Part model, mm, in its own coordinate system. Give positions to 0.01 mm unless a question says otherwise; leave off trailing zeros. Write each loop counter-clockwise with the first axis right and the second up, starting at its lowest first coordinate (ties: lowest second). Pieces come first, ordered by that corner, then holes. Notation, with made-up numbers: M 36.5,37.25 L 84.5,37.25 A23 ccw 84.5,68.25 Z; hole C 75.25,-2 d10. An arc over 180 degrees is marked long. Use CSV: the item, a comma, the result in double quotes. Start each with the question number.
Item 1: Cut at A-A (z = 46). List the corners of the cut face in (x, y), then the cut area to 3 significant figures.
Item 2: Mould opens along Y. For faces 1 (the flat face through (0, -1.23, 47.34)), 2 (the flat face through (5, -5.2, 47)), 3 (the cylindrical face through (4.93, -0.496, 44.425)) say: released by +Y, released by -Y, zero draft, split by the parting line, or undercut.
Item 3: Cut at C-C (x = 4.5). List the corners of the cut face in (y, z).
Item 4: Pin check, flat tip, straight feed: pin 1 (5 mm diameter, centred on x = 3.5, y = 3, fed in from -Z). Stop position of the tip, or through.
Item 5: Cut at D-D (x = 9.25). List the corners of the cut face in (y, z), then the cut area to 3 significant figures.
Item 6: Drill centre lines: line 1 (Y direction, x = 7.5, z = 46); line 2 (Z direction, x = 2.75, y = -1.5); line 3 (Z direction, x = 6.75, y = 0). Where is each one in solid material? Low to high. Write a range as [from, to].
Item 7: Cut at B-B (y = 0). List the corners of the cut face in (x, z), then the cut area to 3 significant figures.
Autodesk Inventor part; units mm, degrees
ref_plane "YZ Plane" through (0, 0, 0) normal (1, 0, 0) x (0, 1, 0)
ref_plane "XZ Plane" through (0, 0, 0) normal (0, 1, 0) x (-1, 0, 0)
ref_plane "XY Plane" through (0, 0, 0) normal (0, 0, 1) x (1, 0, 0)
sketch "Sketch1" plane through (0, 0, 0) normal (1, 0, 0) x (0, 1, 0)
  circle A0 centre (0, 0) radius 54
  circle A1 centre (0, 46) radius 1
  circle A2 centre (0, 46) radius 5.5
  line L0 (5.2, 40.5) -> (-5.2, 40.5)
  arc A3 (5.2, 53.749) -> (-5.2, 53.749) centre (0, 0) ccw
  line L1 (5.2, 53.749) -> (5.2, 40.5)
  line L2 (-5.2, 53.749) -> (-5.2, 40.5)
  circle A4 centre (0, 46) radius 5.2
  dimension "d0" = 108
  dimension "d1" = 46
  dimension "d2" = 2
  dimension "d3" = 11
  dimension "d23" = 10.4
  dimension "d24" = 0
extrude "Extrusion1" add sketch "Sketch1" along normal blind 10 contours L1 A2 L2 A0 | L1 A4 L2 A2 | A4 | L1 A2 L2 A4 | A2 L0 L2 | L1 L0 A2 | A1
sketch "Sketch2" plane through (10, 0, 0) normal (1, 0, 0) x (0, 0, -1)
  circle A0 centre (0, 0) radius 54
  point P0 (-46, 0)
  dimension "d15" = 46
hole "Hole2" at (10, 0, 46) direction (-1, 0, 0) diameter 3.302 end through all
sketch "Sketch3" plane through (0, -5.2, 40.5) normal (0, -1, 0) x (1, 0, 0)
  line L0 (0, 0) -> (10, 0)
  line L1 (0, 0) -> (10, 0)
  line L2 (10.0706, -0.8811) -> (0, 0)
  line L3 (10, 13.249) -> (10, 0)
  line L4 (10, 0) -> (10, -0.8749)
  point P0 (0, -40.5)
  dimension "d25" = 5
extrude "Extrusion2" add sketch "Sketch3" against normal up to surface (10.4 mm away)
properties part number "32110_Lock Wedge_V1" material "Acetal Resin, White"
Worked answers:
1,outline,"M 0,-5.2 L 10,-5.2 L 10,-1.65 L 0,-1.65 Z; M 0,1.65 L 10,1.65 L 10,5.2 L 0,5.2 Z"
1,area,"71.0 mm^2"
2,face 1,"zero draft"
2,face 2,"released by -Y"
2,face 3,"undercut"
3,outline,"M -5.2,40.11 L 5.2,40.11 L 5.2,53.75 A54 ccw -5.2,53.75 Z; hole C 0,46 d3.3"
4,pin 1,"stops at z = 39.98"
5,outline,"M -5.2,39.69 L 5.2,39.69 L 5.2,53.75 A54 ccw -5.2,53.75 Z; hole C 0,46 d3.3"
5,area,"139 mm^2"
6,line 1,"y = [-5.2, -1.65], [1.65, 5.2]"
6,line 2,"z = [40.26, 45.31], [46.69, 53.98]"
6,line 3,"z = [39.91, 44.35], [47.65, 54]"
7,outline,"M 0,40.5 L 10,39.63 L 10,44.35 L 0,44.35 Z; M 0,47.65 L 10,47.65 L 10,54 L 0,54 Z"
7,area,"106 mm^2"
